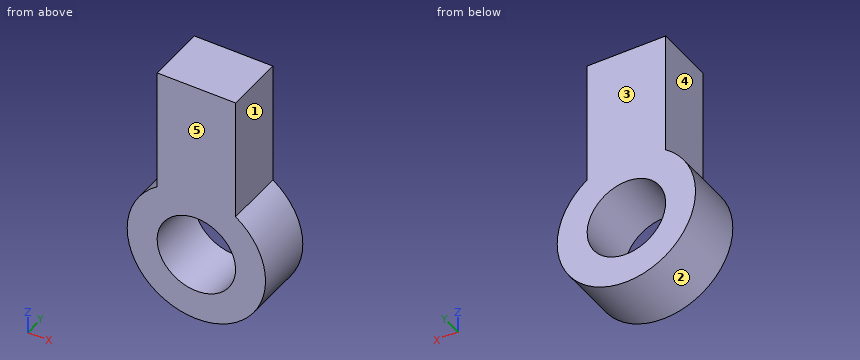
```python
from build123d import *

# Parameters (mm, degrees)
SKETCH1_R           = 5.8674
SKETCH1_R_2         = 3.3274
BOSS_EXTRUDE1_DEPTH = 5.08
BOSS_EXTRUDE2_DEPTH = 5.08


with BuildPart() as part:
    # Sketch1 → Boss-Extrude1 (new body)
    with BuildSketch(Plane(origin=(0, 0, 0), x_dir=(-1, 0, 0), z_dir=(0, 1, 0))):
        with Locations(Location((0, 0, 0), (0, 0, 90))):
            Circle(SKETCH1_R)
        with Locations(Location((0, 0, 0), (0, 0, 90))):
            Circle(SKETCH1_R_2, mode=Mode.SUBTRACT)
    extrude(amount=BOSS_EXTRUDE1_DEPTH)

    # Sketch2 → Boss-Extrude2 (add)
    with BuildSketch(Plane.XZ):
        with BuildLine():
            Line((-3.3274, 0), (-3.3274, 15.24))
            Line((-3.3274, 15.24), (3.3274, 15.24))
            Line((3.3274, 15.24), (3.3274, 0))
            ThreePointArc((3.3274, 0), (0, 3.3274), (-3.3274, 0))
        make_face()
    extrude(amount=-BOSS_EXTRUDE2_DEPTH)


solid = part.part
```
Work out the finished part from the listing and answer in its coordinate system (mm). Face numbers are marked on the shaded views. A direction names the side the tool comes from. Give positions to 0.01 mm unless a question says otherwise; leave off trailing zeros. Loops run counter-clockwise (first coordinate to the right, second up) from the corner with the lowest first, then second, coordinate; pieces in that order, holes last. Notation, with made-up numbers: (50, 79) -> (71, 79) arc R24 ccw to (71, 91) -> close; hole circle Ø6 at (7.5, 86). An arc over 180 degrees is marked (long way). Write item = value, one per line. Start each with the question number.
(1) The mould has two halves that part along Y. Classify the marked faces 3, 4 and 5: +Y half, -Y half, draft (parallel to the pull), parting line (faces both ways), or undercut.
(2) Find section D-D on z = 12. Give the vertices of the cut face in (x, y).
(3) Which of the six approach directions +Z, -Z, +X, -X, +Y, -Y give full straight-line access (tool end or side, diameter ignored) to the marked faces 1 and 2?
(4) Find section A-A on z = 0. Give the vertices of the cut face in (x, y).
(5) Find the intervals of material crossed by probe 1 along X at (y, z) = (1.3, 0); probe 2 along X at (y, z) = (4.25, 14.25); probe 3 along X at (y, z) = (1.35, -2), in increasing order. Write a range as from..to.
(6) Given pin 1 Ø2 at (y, z) = (2, 6) entering from +X; pin 2 Ø3 at (y, z) = (2.5, 8.5) entering from -X, each flat-ended and moving along its own axis, determine where each tip first touches the part or whether it passes through.
(7) Find section C-C on y = 1.9. Give the vertices of the cut face in (x, z), and give its area (3 significant figures).
(8) Find section B-B on x = 0. Give the vertices of the cut face in (y, z).
From the geometry:
q1.face_3 = +Y half
q1.face_4 = draft
q1.face_5 = -Y half
q2.outline = (-3.33, 0) -> (3.33, 0) -> (3.33, 5.08) -> (-3.33, 5.08) -> close
q3.face_1 = +Z, +X, +Y, -Y
q3.face_2 = +Y, -Y
q4.outline = (-5.87, 0) -> (-3.33, 0) -> (-3.33, 5.08) -> (-5.87, 5.08) -> close; (3.33, 0) -> (5.87, 0) -> (5.87, 5.08) -> (3.33, 5.08) -> close
q5.probe_1 = -5.87..-3.33, 3.33..5.87
q5.probe_2 = -3.33..3.33
q5.probe_3 = -5.52..-2.66, 2.66..5.52
q6.pin_1 = 3.33
q6.pin_2 = -3.33
q7.outline = (-3.33, 4.83) arc R5.87 ccw (long way) to (3.33, 4.83) -> (3.33, 15.24) -> (-3.33, 15.24) -> close; hole circle Ø6.65 at (0, 0)
q7.area = 138 mm^2
q8.outline = (0, -5.87) -> (5.08, -5.87) -> (5.08, -3.33) -> (0, -3.33) -> close; (0, 3.33) -> (5.08, 3.33) -> (5.08, 15.24) -> (0, 15.24) -> close
